Work out the finished part from the listing and answer in its coordinate system (mm). Give positions to 0.01 mm unless a question says otherwise; leave off trailing zeros. Order: outer loops, then holes, each group sorted by start corner. A loop starts at its lowest first (then second) coordinate and runs counter-clockwise, first axis right, second up. Notation, with made-up numbers: M 26,-13.75 L 49,-13.75 A5 ccw 49,-5.75 Z; hole C 68,-1.75 d7. An arc over 180 degrees is marked long. One line per item, written item: value.
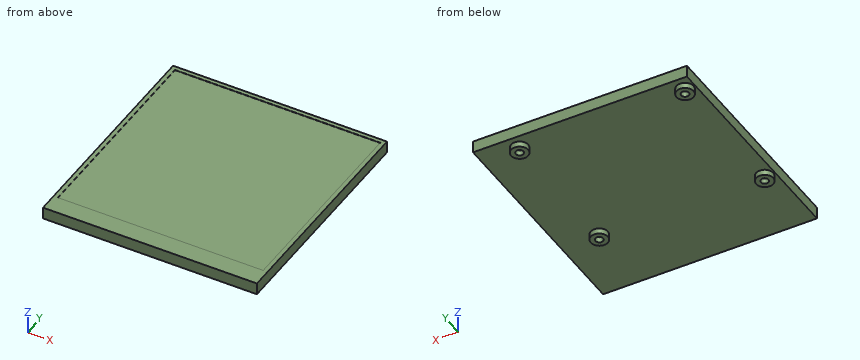
from build123d import *

# Parameters (mm, degrees)
SKETCH1_W           = 75
SKETCH1_H           = 80
BOSS_EXTRUDE1_DEPTH = 4.2
SKETCH2_W           = 72
SKETCH2_H           = 72
CUT_EXTRUDE1_DEPTH  = 0.1
SKETCH3_R           = 3
SKETCH3_R_2         = 1.35
BOSS_EXTRUDE2_DEPTH = 2


with BuildPart() as part:
    # Sketch1 → Boss-Extrude1 (new body)
    with BuildSketch(Plane.XY):
        with Locations((37.5, 40)):
            Rectangle(SKETCH1_W, SKETCH1_H)
    extrude(amount=BOSS_EXTRUDE1_DEPTH)

    # Sketch2 → Cut-Extrude1 (cut)
    with BuildSketch(Plane.XY.offset(4.2)):
        with Locations((37.5, 42.5)):
            Rectangle(SKETCH2_W, SKETCH2_H)
    extrude(amount=-CUT_EXTRUDE1_DEPTH, mode=Mode.SUBTRACT)

    # Sketch3 → Boss-Extrude2 (add)
    with BuildSketch(Plane(origin=(0, 0, 0), x_dir=(-1, 0, 0), z_dir=(0, 0, -1))):
        with Locations((-61.5, 75)):
            Circle(SKETCH3_R)
        with Locations((-61.5, 75)):
            Circle(SKETCH3_R_2, mode=Mode.SUBTRACT)
        with Locations((-3.5, 75)):
            Circle(SKETCH3_R)
        with Locations((-3.5, 75)):
            Circle(SKETCH3_R_2, mode=Mode.SUBTRACT)
        with Locations((-3.5, 26)):
            Circle(SKETCH3_R)
        with Locations((-3.5, 26)):
            Circle(SKETCH3_R_2, mode=Mode.SUBTRACT)
        with Locations((-61.5, 26)):
            Circle(SKETCH3_R)
        with Locations((-61.5, 26)):
            Circle(SKETCH3_R_2, mode=Mode.SUBTRACT)
    extrude(amount=BOSS_EXTRUDE2_DEPTH)


solid = part.part
(1) Section A-A, the plane z = -1 is taken. Give the vertices of the cut face in (x, y), then the cut area to 3 significant figures.
Findings:
outline: C 3.5,26 d6; C 3.5,75 d6; C 61.5,26 d6; C 61.5,75 d6; hole C 3.5,26 d2.7; hole C 3.5,75 d2.7; hole C 61.5,26 d2.7; hole C 61.5,75 d2.7
area: 90.2 mm^2
(2) Section B-B, the plane y = 18.5 is taken. Give the vertices of the cut face in (x, z), then the cut area to 3 significant figures.
Findings:
outline: M 0,0 L 75,0 L 75,4.2 L 73.5,4.2 L 73.5,4.1 L 1.5,4.1 L 1.5,4.2 L 0,4.2 Z
area: 308 mm^2
(3) Given P1, Ø10, axis at x = 42.5, y = 33, coming from the +Z side; P2, Ø1, axis at x = 31.5, y = 11.5, coming from the -Z side, each flat-ended and moving along its own axis, determine where each tip first touches the part or whether it passes through.
Findings:
P1: stops at z = 4.1
P2: stops at z = 0
(4) Section C-C, the plane x = 3.5 is taken. Give the vertices of the cut face in (y, z).
Findings:
outline: M 0,0 L 23,0 L 23,-2 L 24.65,-2 L 24.65,0 L 27.35,0 L 27.35,-2 L 29,-2 L 29,0 L 72,0 L 72,-2 L 73.65,-2 L 73.65,0 L 76.35,0 L 76.35,-2 L 78,-2 L 78,0 L 80,0 L 80,4.2 L 78.5,4.2 L 78.5,4.1 L 6.5,4.1 L 6.5,4.2 L 0,4.2 Z
(5) Find the intervals of material crossed by probe 1 along Y at (x, z) = (3.5, -0.5); probe 2 along Z at (x, y) = (42, 14), in increasing order. Write a range as from..to.
Findings:
probe 1: y = 23..24.65, 27.35..29, 72..73.65, 76.35..78
probe 2: z = 0..4.1
(6) Section D-D, the plane x = 43.5 is taken. Give the vertices of the cut face in (y, z).
Findings:
outline: M 0,0 L 80,0 L 80,4.2 L 78.5,4.2 L 78.5,4.1 L 6.5,4.1 L 6.5,4.2 L 0,4.2 Z
